Work out the finished part from the listing and answer in its coordinate system (mm). A direction names the side the tool comes from. Round coordinates to 2 decimals unless told otherwise and drop trailing zeros. Write each loop counter-clockwise with the first axis right and the second up, starting at its lowest first coordinate (ties: lowest second). Pieces come first, ordered by that corner, then holes. Notation, with made-up numbers: (81, 75) - (94, 75) arc R12 cw to (94, 91) - close; hole circle Ø2 at (28, 35). An arc over 180 degrees is marked (long way). Answer as a JSON object with one key per item and string values.
```python
from build123d import *

# Parameters (mm, degrees)
F0_W           = 76.2
F0_H           = 63.5
F1_DEPTH       = 25.4
F3_D           = 6.7564
F3_CBORE_D     = 11.1125
F3_CBORE_DEPTH = 6.35
F4_R           = 1.5875


with BuildPart() as f1:
    # F0 (on Front) → F1 (new body)
    with BuildSketch(Plane.XZ):
        Rectangle(F0_W, F0_H)
    extrude(amount=F1_DEPTH)

    # F3 (through all)
    with Locations(Plane.XZ.offset(25.4)):
        with Locations((-22.225, 22.225), (22.225, 22.225), (22.225, -22.225), (-22.225, -22.225)):
            CounterBoreHole(F3_D / 2, F3_CBORE_D / 2, F3_CBORE_DEPTH)

    # F4
    f4_edges = [f1.edges().sort_by_distance(p)[0] for p in [
        (0, -25.4, 31.75),
        (38.1, -25.4, 0),
        (0, -25.4, -31.75),
        (-38.1, -25.4, 0),
    ]]
    fillet(f4_edges, radius=F4_R)


solid = f1.part
```
Item 1: Each of these flat-tipped pins is pushed along its axis until it touches: P1, Ø6.5, axis at x = -22.225, z = 22.225, coming from the +Y side; P2, Ø5.5, axis at x = 23.5, z = 24.5, coming from the -Y side. Where does it stop, or does it pass through?
Results found:
{"P1": "through", "P2": "y = -19.05"}
Item 2: For faces 4 (the flat face through (-1, -12, -31.75)), 5 (the cylindrical face through (-27.776, -22.269, -21.981)), determine the directions among +Z, -Z, +X, -X, +Y, -Y from which every point of the face is accessible in a straight line to the end or side of a thin tool.
Results found:
{"face 4": "-Z, +X, -X, +Y, -Y", "face 5": "-Y"}
Item 3: A cutting plane is placed at B-B (y = -15.5). Write down the section's boundary in (x, z) (3 decimals).
Results found:
{"outline": "(-38.1, -31.75) - (38.1, -31.75) - (38.1, 31.75) - (-38.1, 31.75) - close; hole circle Ø6.756 at (-22.225, -22.225); hole circle Ø6.756 at (-22.225, 22.225); hole circle Ø6.756 at (22.225, -22.225); hole circle Ø6.756 at (22.225, 22.225)"}
Item 4: Determine the mould class of faces 1 (the flat face through (38.1, -12, 0)), 2 (the flat face through (25, -19.05, 20)), 3 (the flat face through (-1, -25.4, 0)) for opening direction X: pulls with the +X half, pulls with the -X half, needs draft (parallel to the pull), parting line crosses it, or undercut.
Results found:
{"face 1": "pulls with the +X half", "face 2": "undercut", "face 3": "needs draft"}
Item 5: A cutting plane is placed at A-A (x = 24.5). Give the number of separate pieces and of enclosed holes in the cut face, and give its area (3 significant figures).
Results found:
{"separate pieces": "3", "enclosed holes": "0", "area": "1,290 mm²"}
Item 6: Consider line 1 along X through (y, z) = (-9.25, 22.5); line 2 along X through (y, z) = (-4, 20); line 3 along Y through (x, z) = (20, -19.5). Determine where each line is inside the solid, lowest interval first.
Results found:
{"line 1": "-38.1 to -25.59, -18.86 to 18.86, 25.59 to 38.1", "line 2": "-38.1 to -24.77, -19.68 to 19.68, 24.77 to 38.1", "line 3": "-19.05 to 0"}
